Geometry: final body of the model. Coordinates: model frame, mm. Face numbers are marked on the shaded views. A direction names the side the tool comes from. Give positions to 0.01 mm unless a question says otherwise; leave off trailing zeros. Order: outer loops, then holes, each group sorted by start corner. A loop starts at its lowest first (then second) coordinate and runs counter-clockwise, first axis right, second up. Notation, with made-up numbers: (-29, 87) -> (-6, 87) arc R13 ccw to (-6, 104) -> close; hole circle Ø7 at (66, 31). An arc over 180 degrees is marked (long way). Answer in a Markdown table with one row per item. Add a question column.
Q1. Contact query for flat-ended pins moving along their axis: P1, Ø11, axis at y = 59, z = -2, coming from the +X side (3 decimals); P2, Ø10, axis at x = -2.5, y = 26, coming from the +Z side (3 decimals); P3, Ø12, axis at y = 58, z = -8, coming from the +X side. Output: stop coordinate, or through.
Q2. Cut plane A-A on y = 59.5. Return the cut outline in (x, z), and give its area (3 significant figures).
Q3. Cut plane C-C on y = 72.5. Return the cut outline in (x, z), and give its area (3 significant figures).
Q4. Cut plane B-B on y = 9. Return the cut outline in (x, z) (3 decimals), and give its area (3 significant figures).
Q5. Set-up query: the marked faces 1, 2, 3 and 4. Return all of +Z, -Z, +X, -X, +Y, -Y with unobstructed straight access to the full face (end or side cutting, diameter ignored); none if empty.
Q6. Line query: line 1 along Y through (x, z) = (17, 11.5); line 2 along Y through (x, z) = (-10, -3.5); line 3 along X through (y, z) = (28, -1). Output: solid intervals per line, ascending. Write a range as from..to.
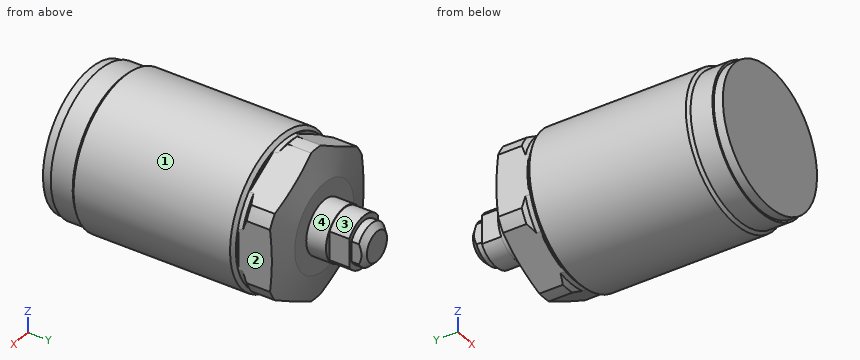
from build123d import *

# Parameters (mm, degrees)
SKETCH2_OUTSIDE_W       = 66.07
SKETCH2_OUTSIDE_H       = 66.07
CUT_EXTRUDE1_DEPTH      = 12
CHAMFER1_SIZE           = 1.754
SKETCH5_W               = 2.285
SKETCH5_H               = 3.988
CUT_EXTRUDE2_DEPTH      = 23.5
CUT_EXTRUDE2_DEPTH_BACK = 23.5
SKETCH6_W               = 1.575
SKETCH6_H               = 6.02
CUT_EXTRUDE3_DEPTH      = 23.5
CUT_EXTRUDE3_DEPTH_BACK = 23.5


with BuildPart() as part:
    # Sketch1 → Revolve1 (revolve)
    with BuildSketch(Plane.XY, mode=Mode.PRIVATE) as revolve1_sk:
        Polygon((-21.575, 0), (-21, 0), (-21, -2.75), (0, -2.75), (0, 68.25), (-13.125, 68.25), (-22.5, 65.737976321), (-22.5, 58.625), (-21.375, 57.5), (-21.375, 56), (-22.425, 54.95), (-22.425, 7.5), (-21.575, 6.65), align=None)
    revolve(revolve1_sk.sketch.rotate(Axis((0, 0, 0), (0, -1, 0)), 270), axis=Axis((0, 0, 0), (0, -1, 0)))  # turned: the seam where the file's is

    # Sketch2 outside → Cut-Extrude1 (cut)
    with BuildSketch(Plane(origin=(0, 68.25, 0), x_dir=(1, 0, 0), z_dir=(0, 1, 0))):
        Rectangle(SKETCH2_OUTSIDE_W, SKETCH2_OUTSIDE_H)
        Polygon((0, 23.625173015), (-20.46, 11.812586508), (-20.46, -11.812586508), (0, -23.625173015), (20.46, -11.812586508), (20.46, 11.812586508), align=None, mode=Mode.SUBTRACT)
    extrude(amount=-CUT_EXTRUDE1_DEPTH, mode=Mode.SUBTRACT)

    # Sketch4 → Revolve2 (revolve)
    with BuildSketch(Plane.XY, mode=Mode.PRIVATE) as revolve2_sk:
        Polygon((0, 84.25), (-6.25, 84.25), (-6.25, 80.262), (-7.745, 80.262), (-7.745, 74.242), (-8, 74.242), (-8, 68.25), (0, 68.25), align=None)
    revolve(revolve2_sk.sketch.rotate(Axis((0, 0, 0), (0, 1, 0)), 90), axis=Axis((0, 0, 0), (0, 1, 0)))  # turned: the seam where the file's is

    # Chamfer1
    chamfer1_edges = [part.edges().sort_by_distance(p)[0] for p in [
        (0, 84.25, -6.25),
    ]]
    chamfer(chamfer1_edges, length=CHAMFER1_SIZE)

    # Sketch5 → Cut-Extrude2 (cut, two sides)
    with BuildSketch(Plane.XY) as cut_extrude2_sk:
        with Locations((-6.6025, 82.256)):
            Rectangle(SKETCH5_W, SKETCH5_H)
        with Locations((6.6025, 82.256)):
            Rectangle(SKETCH5_W, SKETCH5_H)
    extrude(amount=CUT_EXTRUDE2_DEPTH, mode=Mode.SUBTRACT)
    extrude(cut_extrude2_sk.sketch, amount=-CUT_EXTRUDE2_DEPTH_BACK, mode=Mode.SUBTRACT)

    # Sketch6 → Cut-Extrude3 (cut, two sides)
    with BuildSketch(Plane.XY) as cut_extrude3_sk:
        with Locations((-7.2125, 77.252)):
            Rectangle(SKETCH6_W, SKETCH6_H)
        with Locations((7.2125, 77.252)):
            Rectangle(SKETCH6_W, SKETCH6_H)
    extrude(amount=CUT_EXTRUDE3_DEPTH, mode=Mode.SUBTRACT)
    extrude(cut_extrude3_sk.sketch, amount=-CUT_EXTRUDE3_DEPTH_BACK, mode=Mode.SUBTRACT)


solid = part.part
Completed:
| question | item | result |
|---|---|---|
| 1 | P1 | stops at x = 22.425 |
| 1 | P2 | stops at z = 22.425 |
| 1 | P3 | stops at x = 22.25 |
| 2 | outline | (-20.46, -9.36) arc R22.5 ccw to (-18.34, -13.04) -> (-2.12, -22.4) arc R22.5 ccw to (2.12, -22.4) -> (18.34, -13.04) arc R22.5 ccw to (20.46, -9.36) -> (20.46, 9.36) arc R22.5 ccw to (18.34, 13.04) -> (2.12, 22.4) arc R22.5 ccw to (-2.12, 22.4) -> (-18.34, 13.04) arc R22.5 ccw to (-20.46, 9.36) -> close |
| 2 | area | 1,440 mm² |
| 3 | outline | circle Ø16 at (0, 0) |
| 3 | area | 201 mm² |
| 4 | outline | circle Ø44.85 at (0, 0) |
| 4 | area | 1,580 mm² |
| 5 | face 1 | -Y |
| 5 | face 2 | +Z, -Z, +X, +Y |
| 5 | face 3 | +Z, +Y |
| 5 | face 4 | +Y |
| 6 | line 1 | y = -2.75..66.27 |
| 6 | line 2 | y = -2.75..68.25 |
| 6 | line 3 | x = -22.4..22.4 |
